Part model, mm, in its own coordinate system. A direction names the side the tool comes from. Give positions to 0.01 mm unless a question says otherwise; leave off trailing zeros. Order: outer loops, then holes, each group sorted by start corner. A loop starts at its lowest first (then second) coordinate and runs counter-clockwise, first axis right, second up. Notation, with made-up numbers: (82.25, -33) - (102.25, -33) arc R12 cw to (102.25, -21) - close; hole circle Ø9 at (-25.75, 79). An arc over 180 degrees is marked (long way). Use one line per item in the form item = value. Start each with the question number.
1. Tool access for faces 1 (the face through (15, 0, -23)), 2 (the face through (10, 2, -29.5)), 3 (the face through (13, 2, -11)): list every direction of +Z, -Z, +X, -X, +Y, -Y with a clear straight run to the whole face (end or side of a thin tool).
2. Band-saw the part on B-B, the plane x = 9.75. State how many separate pieces and enclosed holes the cut face has, plus the area to 3 significant figures.
3. Pull direction Z, two halves, no side cores. Call faces 4 (the face through (24.92, 1.61, -0.45)), 5 (the face through (13.098, 1.61, -28.787)), 6 (the face through (0, 2, -22)): +Z half, -Z half, draft (parallel to the pull), parting line (faces both ways), or undercut.
4. Drill centre lines: line 1 (Z direction, x = 8.75, y = 2.3); line 2 (Z direction, x = 17.9, y = 1.25) (3 decimals); line 3 (Z direction, x = 9.75, y = 0.6). Where is each one in solid material? Low to high.
5. Band-saw the part on D-D, the plane z = -21. List the corners of the cut face in (x, y) (3 decimals).
6. Pin check, flat tips, straight feed: P1, Ø3, axis at x = 17.9, z = -26.975, coming from the -Y side; P2, Ø4.5, axis at x = 16, z = -5, coming from the +Y side. Stop position of each tip, or through.
from build123d import *

# Parameters (mm, degrees)
SKETCH1_W           = 25.4
SKETCH1_H           = 44.45
SKETCH1_R           = 1.2
BOSS_EXTRUDE1_DEPTH = 3.175
CUT_EXTRUDE1_DEPTH  = 4.175
FILLET1_R           = 1.5875
CUT_EXTRUDE2_DEPTH  = 1.5875


with BuildPart() as part:
    # Sketch1 → Boss-Extrude1 (new body)
    with BuildSketch(Plane(origin=(0, 0, 0), x_dir=(1, 0, 0), z_dir=(0, 1, 0))):
        with Locations((12.7, 22.225)):
            Rectangle(SKETCH1_W, SKETCH1_H)
        with Locations((17.9, 17.475)):
            Circle(SKETCH1_R, mode=Mode.SUBTRACT)
        with Locations((17.9, 26.975)):
            Circle(SKETCH1_R, mode=Mode.SUBTRACT)
        with BuildLine():
            Line((5.425, 8.6), (20.425, 8.6))
            ThreePointArc((20.425, 8.6), (22.675, 6.35), (20.425, 4.1))
            Line((20.425, 4.1), (5.425, 4.1))
            ThreePointArc((5.425, 4.1), (3.175, 6.35), (5.425, 8.6))
        make_face(mode=Mode.SUBTRACT)
        with BuildLine():
            Line((5.425, 35.85), (20.425, 35.85))
            ThreePointArc((20.425, 35.85), (22.675, 38.1), (20.425, 40.35))
            Line((20.425, 40.35), (5.425, 40.35))
            ThreePointArc((5.425, 40.35), (3.175, 38.1), (5.425, 35.85))
        make_face(mode=Mode.SUBTRACT)
    extrude(amount=BOSS_EXTRUDE1_DEPTH)

    # Sketch2 → Cut-Extrude1 (cut, through all)
    with BuildSketch(Plane(origin=(0, 3.175, 0), x_dir=(1, 0, 0), z_dir=(0, 1, 0))):
        with BuildLine():
            Line((11.35, 14.95), (8.85, 14.95))
            ThreePointArc((8.85, 14.95), (7.082233047, 15.682233047), (6.35, 17.45))
            Line((6.35, 17.45), (6.35, 27))
            ThreePointArc((6.35, 27), (7.082233047, 28.767766953), (8.85, 29.5))
            Line((8.85, 29.5), (11.35, 29.5))
            ThreePointArc((11.35, 29.5), (13.117766953, 28.767766953), (13.85, 27))
            Line((13.85, 27), (13.85, 17.45))
            ThreePointArc((13.85, 17.45), (13.117766953, 15.682233047), (11.35, 14.95))
        make_face()
    extrude(amount=-CUT_EXTRUDE1_DEPTH, mode=Mode.SUBTRACT)

    # Fillet1
    fillet1_edges = [part.edges().sort_by_distance(p)[0] for p in [
        (0, 1.5875, -44.45),
        (25.4, 1.5875, -44.45),
        (25.4, 1.5875, 0),
        (0, 1.5875, 0),
    ]]
    fillet(fillet1_edges, radius=FILLET1_R)

    # Sketch3 → Cut-Extrude2 (cut)
    with BuildSketch(Plane(origin=(0, 3.175, 0), x_dir=(1, 0, 0), z_dir=(0, 1, 0))):
        with BuildLine():
            Line((5.425, 33.45), (20.425, 33.45))
            ThreePointArc((20.425, 33.45), (25.075, 38.1), (20.425, 42.75))
            Line((20.425, 42.75), (5.425, 42.75))
            ThreePointArc((5.425, 42.75), (0.775, 38.1), (5.425, 33.45))
        make_face()
        with BuildLine():
            Line((5.425, 1.7), (20.425, 1.7))
            ThreePointArc((20.425, 1.7), (25.075, 6.35), (20.425, 11))
            Line((20.425, 11), (5.425, 11))
            ThreePointArc((5.425, 11), (0.775, 6.35), (5.425, 1.7))
        make_face()
    extrude(amount=-CUT_EXTRUDE2_DEPTH, mode=Mode.SUBTRACT)


solid = part.part
From the geometry:
q1.face_1 = +Z, -Z, +X, -X, -Y
q1.face_2 = +Y, -Y
q1.face_3 = +Y
q2.separate_pieces = 4
q2.enclosed_holes = 0
q2.area = 51.1 mm²
q3.face_4 = +Z half
q3.face_5 = undercut
q3.face_6 = draft
q4.line_1 = -44.45 to -42.75, -33.45 to -29.5, -14.95 to -11, -1.7 to 0
q4.line_2 = -44.45 to -40.35, -35.85 to -28.175, -25.775 to -18.675, -16.275 to -8.6, -4.1 to 0
q4.line_3 = -44.45 to -40.35, -35.85 to -29.5, -14.95 to -8.6, -4.1 to 0
q5.outline = (0, 0) - (6.35, 0) - (6.35, 3.175) - (0, 3.175) - close; (13.85, 0) - (25.4, 0) - (25.4, 3.175) - (13.85, 3.175) - close
q6.P1 = 0
q6.P2 = 1.59
